```python
from build123d import *

# Parameters (mm, degrees)
BOSS_EXTRUDE3_DEPTH = 48
SKETCH4_R           = 2.625
CUT_EXTRUDE2_DEPTH  = 14.608970631
SKETCH5_R           = 2.625
CUT_EXTRUDE3_DEPTH  = 14.608970631
FILLET2_R           = 2.5
CUT_EXTRUDE4_DEPTH  = 12.5
CUT_EXTRUDE6_DEPTH  = 12.5
FILLET3_R           = 1
FILLET4_R           = 1


with BuildPart() as part:
    # Sketch2 → Boss-Extrude3 (new body)
    with BuildSketch(Plane.XY):
        Polygon((0, 2.309401077), (-11, -6.350852961), (11, -6.350852961), align=None)
    extrude(amount=BOSS_EXTRUDE3_DEPTH)

    # Sketch4 → Cut-Extrude2 (cut, through all)
    with BuildSketch(Plane(origin=(-1.12244898, 1.425701685, 0), x_dir=(0.785714286, 0.618589574, 0), z_dir=(-0.618589574, 0.785714286, 0))):
        with Locations((-7.321428571, -24)):
            Circle(SKETCH4_R)
    extrude(amount=-CUT_EXTRUDE2_DEPTH, mode=Mode.SUBTRACT)

    # Sketch5 → Cut-Extrude3 (cut, through all)
    with BuildSketch(Plane(origin=(1.12244898, 1.425701685, 0), x_dir=(0.785714286, -0.618589574, 0), z_dir=(0.618589574, 0.785714286, 0))):
        with Locations((5.321428571, -11.5)):
            Circle(SKETCH5_R)
        with Locations((5.321428571, -36.5)):
            Circle(SKETCH5_R)
    extrude(amount=-CUT_EXTRUDE3_DEPTH, mode=Mode.SUBTRACT)

    # Fillet2
    fillet2_edges = [part.edges().sort_by_distance(p)[0] for p in [
        (0, 2.309401077, 24),
    ]]
    fillet(fillet2_edges, radius=FILLET2_R)

    # Sketch6 → Cut-Extrude4 (cut)
    with BuildSketch(Plane(origin=(-8.156394632, -10.360012601, 0), x_dir=(0.785714286, -0.618589574, 0), z_dir=(0.618589574, 0.785714286, 0))):
        Polygon((7.160320357, -7.200177097), (2.517118598, -7.757561547), (0.678226812, -12.05738445), (3.482536786, -15.799822903), (8.125738545, -15.242438453), (9.96463033, -10.94261555), align=None)
        Polygon((7.160320357, -32.200177097), (2.517118598, -32.757561547), (0.678226812, -37.05738445), (3.482536786, -40.799822903), (8.125738545, -40.242438453), (9.96463033, -35.94261555), align=None)
    extrude(amount=CUT_EXTRUDE4_DEPTH, mode=Mode.SUBTRACT)

    # Sketch7 → Cut-Extrude6 (cut)
    with BuildSketch(Plane(origin=(8.156394632, -10.360012601, 0), x_dir=(0.785714286, 0.618589574, 0), z_dir=(-0.618589574, 0.785714286, 0))):
        Polygon((-7.321428571, -19.32346282), (-11.371428571, -21.66173141), (-11.371428571, -26.33826859), (-7.321428571, -28.67653718), (-3.271428571, -26.33826859), (-3.271428571, -21.66173141), align=None)
    extrude(amount=CUT_EXTRUDE6_DEPTH, mode=Mode.SUBTRACT)

    # Fillet3
    fillet3_edges = [part.edges().sort_by_distance(p)[0] for p in [
        (-6.273236968, -2.629492176, 0),
        (0, 1.627582895, 0),
        (6.273236968, -2.629492176, 0),
    ]]
    fillet(fillet3_edges, radius=FILLET3_R)

    # Fillet4
    fillet4_edges = [part.edges().sort_by_distance(p)[0] for p in [
        (-6.273236968, -2.629492176, 48),
        (0, 1.627582895, 48),
        (6.273236968, -2.629492176, 48),
    ]]
    fillet(fillet4_edges, radius=FILLET4_R)


solid = part.part
```
Could you check a few things on this model? Use its own coordinates, in mm. A direction names the side the tool comes from. Round coordinates to 2 decimals unless told otherwise and drop trailing zeros. Loops run counter-clockwise (first coordinate to the right, second up) from the corner with the lowest first, then second, coordinate; pieces in that order, holes last. Notation, with made-up numbers: (-30.75, 87) - (24.25, 87) arc R17 cw to (24.25, 116) - close; hole circle Ø1 at (37.25, -30.5). An arc over 180 degrees is marked (long way). Answer in a Markdown table with one row per item. Add a question column.
(1) If we section it at B-B (y = -4.5): State how many separate pieces and enclosed holes the cut face has, plus the area to 3 significant figures.
(2) I'm going to push flat-ended pins straight in: pin 1 (6 mm diameter, centred on x = 7.5, z = 41.5, fed in from +Y); pin 2 (1.5 mm diameter, centred on y = -3, z = 29.5, fed in from -X); pin 3 (3 mm diameter, centred on y = -0.5, z = 39.5, fed in from -X). Where does each tip first touch, or does it pass through?
(3) If we section it at A-A (z = 44): Please give me the cut outline in (x, y).
(4) For faces 1 (the face through (2.565, -5.238, 40.587)), 2 (the face through (-0.023, 1.627, 24.322)), which set-ups out of +Z, -Z, +X, -X, +Y, -Y let a thin tool reach every point of the face, with its end or its side?
(5) If we mould it in two halves opening along Z, with no side actions, what happens to faces 3 (the face through (-4.106, -0.923, 23.678)), 4 (the face through (6.03, -2.8, 0.3)), 5 (the face through (-2.98, -3.22, 23.93)), 6 (the face through (-0.634, -4.483, 24.033))? For each: pulls with the +Z half, pulls with the -Z half, needs draft (parallel to the pull), parting line crosses it, or undercut.
(6) I need wall thicknesses on line 1 along Z through (x, y) = (1.75, -3.5); line 2 along Z through (x, y) = (-1.5, -5.5); line 3 along Z through (x, y) = (-1, -4.75). Which ranges of each line are inside material? Lowest first, please.
Model answer:
| question | item | result |
|---|---|---|
| 1 | separate pieces | 1 |
| 1 | enclosed holes | 2 |
| 1 | area | 676 mm² |
| 2 | pin 1 | stops at y = -1.23 |
| 2 | pin 2 | stops at x = -7.7 |
| 2 | pin 3 | stops at x = -5.47 |
| 3 | outline | (-11, -6.35) - (11, -6.35) - (1.55, 1.09) arc R2.5 ccw to (-1.55, 1.09) - close |
| 4 | face 1 | none |
| 4 | face 2 | +Z, -Z, +Y |
| 5 | face 3 | needs draft |
| 5 | face 4 | pulls with the -Z half |
| 5 | face 5 | undercut |
| 5 | face 6 | undercut |
| 6 | line 1 | z = 0 to 7.63, 15.79 to 32.63, 40.79 to 48 |
| 6 | line 2 | z = 0 to 8.44, 14.12 to 20.91, 27.09 to 33.44, 39.12 to 48 |
| 6 | line 3 | z = 0 to 8.61, 14.02 to 21.4, 26.6 to 33.61, 39.02 to 48 |
